from build123d import *


with BuildPart() as part:
    # Sketch1 → Revolve3 (revolve)
    with BuildSketch(Plane.XY, mode=Mode.PRIVATE) as revolve3_sk:
        with BuildLine():
            Line((3.007394206, 42.751736158), (11.652189651, 17.21165811))
            add(Edge.make_bspline(
                [(11.652189651, 17.21165811), (27.092047712, 0.077628738), (8.704480068, -15.086904856)],
                knots=[0, 0, 0, 1, 1, 1], degree=2))
            Line((8.704480068, -15.086904856), (8.704480068, -30.938794565))
            ThreePointArc((8.704480068, -30.938794565), (9.076454456, -31.836820177), (9.974480068, -32.208794565))
            Line((9.974480068, -32.208794565), (24.13, -32.208794565))
            ThreePointArc((24.13, -32.208794565), (25.028025612, -32.580768953), (25.4, -33.478794565))
            Line((25.4, -33.478794565), (25.4, -40.463794565))
            ThreePointArc((25.4, -40.463794565), (25.028025612, -41.361820177), (24.13, -41.733794565))
            Line((24.13, -41.733794565), (0, -41.733794565))
            Line((0, -41.733794565), (0, 44.908794565))
            ThreePointArc((0, 44.908794565), (1.850494588, 44.313774173), (3.007394206, 42.751736158))
        make_face()
    revolve(revolve3_sk.sketch.rotate(Axis((0, 44.908794565, 0), (0, -1, 0)), 180), axis=Axis((0, 44.908794565, 0), (0, -1, 0)))


solid = part.part
CAD build for the part. Positions are in the model's coordinates, mm. A direction names the side the tool comes from. Coordinates: 2 decimals unless noted, no trailing zeros. Loops run counter-clockwise (first coordinate to the right, second up) from the corner with the lowest first, then second, coordinate; pieces in that order, holes last. Notation, with made-up numbers: (-17.5, 36) -> (5.5, 36) arc R21 ccw to (5.5, 72) -> close; hole circle Ø7 at (43.5, -29.75). An arc over 180 degrees is marked (long way). One line per item, written item: value.
1. Slice it at A-A on y = -19. Write the cut outline in (x, z).
Answers:
outline: circle Ø17.41 at (0, 0)
2. Slice it at B-B on y = 35.5. Write the cut outline in (x, z), and give its area (3 significant figures).
Answers:
outline: circle Ø10.92 at (0, 0)
area: 93.7 mm^2
3. Pull direction Y, two halves, no side cores. Call faces 1 (the face through (5.102, 32.641, 3.912)), 2 (the face through (0, -41.734, 0)), 3 (the face through (-0.3, -32.209, 10.4)): pulls with the +Y half, pulls with the -Y half, needs draft (parallel to the pull), parting line crosses it, or undercut.
Answers:
face 1: pulls with the +Y half
face 2: pulls with the -Y half
face 3: undercut
4. Flat gauge pins, fed straight in: P1, Ø12, axis at x = 7, y = -20.5, coming from the +Z side; P2, Ø8, axis at x = 4.5, y = 20, coming from the +Z side; P3, Ø12, axis at y = -11, z = 0, coming from the -X side. Where does each tip first touch, or does it go through?
Answers:
P1: stops at z = 8.65
P2: stops at z = 12.11
P3: stops at x = -17.09
5. Which spindle directions (+Z, -Z, +X, -X, +Y, -Y) get a long thin tool onto all of the face, cutting with end or side? Do faces 4 (the face through (6.4, -23.1, -5.9)), 5 (the face through (-11.721, -37.02, 22.534)). Say none if no direction does.
Answers:
face 4: none
face 5: +Y, -Y
6. Drill centre lines: line 1 (Y direction, x = -3, z = 21); line 2 (Y direction, x = 11.5, z = -2); line 3 (Y direction, x = 1, z = 15). Where is each one in solid material? Low to high. Write a range as [from, to].
Answers:
line 1: y = [-41.73, -32.21]
line 2: y = [-41.73, -32.21], [-12.41, 17.19]
line 3: y = [-41.73, -32.21], [-8.49, 12.88]
